Autodesk Inventor part; units mm, degrees
ref_plane "YZ Plane" through (0, 0, 0) normal (1, 0, 0) x (0, 1, 0)
ref_plane "XZ Plane" through (0, 0, 0) normal (0, 1, 0) x (-1, 0, 0)
ref_plane "XY Plane" through (0, 0, 0) normal (0, 0, 1) x (1, 0, 0)
sketch "Sketch1" plane through (0, 0, 0) normal (0, 0, 1) x (1, 0, 0)
  line L0 (6.4658, -12.7) -> (12.7, -12.7)
  arc A0 (-6.4658, -12.7) -> (6.4658, -12.7) centre (0, 0) ccw
  line L1 (-12.7, -12.7) -> (-6.4658, -12.7)
  line L2 (-12.7, -6.4658) -> (-12.7, -12.7)
  arc A1 (-12.7, 6.4658) -> (-12.7, -6.4658) centre (0, 0) ccw
  line L3 (-12.7, 12.7) -> (-12.7, 6.4658)
  line L4 (-6.4658, 12.7) -> (-12.7, 12.7)
  arc A2 (6.4658, 12.7) -> (-6.4658, 12.7) centre (0, 0) ccw
  line L5 (12.7, 12.7) -> (6.4658, 12.7)
  line L6 (12.7, 6.4658) -> (12.7, 12.7)
  arc A3 (12.7, -6.4658) -> (12.7, 6.4658) centre (0, 0) ccw
  line L7 (12.7, -12.7) -> (12.7, -6.4658)
  arc A4 (22.4506, 22.4506) -> (11.1037, -29.7451) centre (0, 0) ccw
  line L8 (53.8815, -8.9803) -> (157.065, -121.1361)
  line L9 (157.065, -121.1361) -> (447.7579, -29.481)
  line L10 (157.065, -121.1361) -> (461.865, -121.1361) construction
  circle A5 centre (463.0337, -77.9298) radius 50.8
  circle A6 centre (419.3415, -191.752) radius 50.8
  line L11 (463.0337, -77.9298) -> (419.3415, -191.752)
  line L12 (463.0337, -77.9298) -> (584.9537, -77.9298) construction
  arc A7 (-31.41, -4.6344) -> (323.0536, -260.3138) centre (270.1256, 39.8556) ccw
  line L13 (428.1628, -241.7802) -> (323.0536, -260.3138)
  line L14 (428.1628, -241.7802) -> (534.8936, -241.7802) construction
  line L15 (510.4596, -96.1349) -> (466.7674, -209.9571)
  circle A8 centre (0, -19.05) radius 2
  circle A9 centre (19.05, 0) radius 2
  circle A10 centre (-19.05, 0) radius 2
  circle A11 centre (0, 19.05) radius 2
  line L16 (22.4506, 22.4506) -> (53.8815, -8.9803)
  line L17 (52.7468, -14.1998) -> (11.1037, -29.7451)
  arc A12 (52.7468, -14.1998) -> (53.8815, -8.9803) centre (51.6365, -11.2253) ccw
  circle A13 centre (0, -19.05) radius 2.735
  circle A14 centre (-19.05, 0) radius 2.735
  circle A15 centre (0, 19.05) radius 2.735
  circle A16 centre (19.05, 0) radius 2.735
  circle A17 centre (463.0337, -77.9298) radius 25.4
  circle A18 centre (419.3415, -191.752) radius 25.4
  point P0 (50.8347, -14.9136)
  point P1 (54.0605, -9.1748)
  dimension "d0" = 152.4
  dimension "d1" = 304.8
  dimension "d2" = 17.5
  dimension "d3" = 101.6
  dimension "d4" = 101.6
  dimension "d5" = 121.92
  dimension "d6" = 111
  dimension "d7" = 609.6
  dimension "d9" = 170
  dimension "d10" = 4
  dimension "d11" = 4
  dimension "d12" = 4
  dimension "d13" = 4
  dimension "d16" = 50.8
  dimension "d17" = 50.8
extrude "Extrusion1" add sketch "Sketch1" along normal blind 3.175 contours L16 L8 L9 A5 L11 A6 L13 A7 A4 | A6 | A5 | A6 L11 A5 L15 | A13 | A14 | A15 | A16
fillet "Fillet1" radius 203.2 1 edges at (157.065, -121.1361, 1.5875)
properties part number "WhipperArm" material "MDF Medium Density Fiberboard"
The listing builds one solid part. Answer for the finished solid, in the listing's coordinates (mm). A direction names the side the tool comes from. Give positions to 0.01 mm unless a question says otherwise; leave off trailing zeros. Order: outer loops, then holes, each group sorted by start corner. A loop starts at its lowest first (then second) coordinate and runs counter-clockwise, first axis right, second up. Notation, with made-up numbers: (-17, -4) -> (41, -4) arc R6 cw to (41, 5) -> close; hole circle Ø3 at (-23, -4.5). An arc over 180 degrees is marked (long way). Put each result on its own line as item: value.
Item 1: Straight lines are drawn through the part: line 1 (Y direction, x = 19.05, z = 1.15); line 2 (X direction, y = -235, z = 2.55); line 3 (Y direction, x = 182, z = 1.7). For each, find the intervals that lie inside material, in ascending order.
Established:
line 1: y = -132.96 to -2, 2 to 25.4
line 2: x = 138.38 to 445.99
line 3: y = -251.93 to -88.27
Item 2: For a pull along Y with two mould halves and no side action, classify faces 3 (the face through (451.936, -230.717, 1.565)), 4 (the face through (237, -147, 0)), 5 (the face through (487.26, -85.56, 1.57)), 6 (the face through (165.2, -84.406, 1.61)) as released by +Y, released by -Y, zero draft, split by the parting line, or undercut.
Established:
face 3: released by -Y
face 4: zero draft
face 5: undercut
face 6: released by +Y
Item 3: For faces 1 (the face through (362.83, -56.26, 1.57)), 2 (the face through (393.966, -192.869, 1.565)), determine the directions among +Z, -Z, +X, -X, +Y, -Y from which every point of the face is accessible in a straight line to the end or side of a thin tool.
Established:
face 1: +Z, -Z, +Y
face 2: +Z, -Z
Item 4: A cutting plane is placed at D-D on x = 115.5. Give the vertices of the cut face in (y, z) (3 decimals), plus the area to 3 significant figures.
Established:
outline: (-222.811, 0) -> (-63.275, 0) -> (-63.275, 3.175) -> (-222.811, 3.175) -> close
area: 507 mm^2
Item 5: A cutting plane is placed at A-A on x = 406. Give the vertices of the cut face in (y, z) (3 decimals).
Established:
outline: (-245.688, 0) -> (-213.366, 0) -> (-213.366, 3.175) -> (-245.688, 3.175) -> close; (-170.138, 0) -> (-42.647, 0) -> (-42.647, 3.175) -> (-170.138, 3.175) -> close
Item 6: A cutting plane is placed at C-C on y = -114.5. Give the vertices of the cut face in (x, z) (3 decimals).
Established:
outline: (7.3, 0) -> (503.41, 0) -> (503.41, 3.175) -> (7.3, 3.175) -> close
Item 7: A cutting plane is placed at B-B on z = 1.3. Give the vertices of the cut face in (x, y).
Established:
outline: (-31.41, -4.63) arc R304.8 ccw to (323.05, -260.31) -> (428.16, -241.78) arc R50.8 ccw to (466.77, -209.96) -> (510.46, -96.13) arc R50.8 ccw to (447.76, -29.48) -> (280.26, -82.29) arc R203.2 cw to (69.61, -26.08) -> (53.88, -8.98) -> (22.45, 22.45) arc R31.75 ccw to start; hole circle Ø4 at (-19.05, 0); hole (-12.7, -12.7) -> (-6.47, -12.7) arc R14.25 ccw to (6.47, -12.7) -> (12.7, -12.7) -> (12.7, -6.47) arc R14.25 ccw to (12.7, 6.47) -> (12.7, 12.7) -> (6.47, 12.7) arc R14.25 ccw to (-6.47, 12.7) -> (-12.7, 12.7) -> (-12.7, 6.47) arc R14.25 ccw to (-12.7, -6.47) -> close; hole circle Ø4 at (0, -19.05); hole circle Ø4 at (0, 19.05); hole circle Ø4 at (19.05, 0); hole circle Ø50.8 at (419.34, -191.75); hole circle Ø50.8 at (463.03, -77.93)
Item 8: Given P1, Ø1.5, axis at y = -107, z = 1, coming from the +X side; P2, Ø1.6, axis at x = 9, z = 1.5, coming from the -Y side; P3, Ø3, axis at x = 0, y = -19.05, coming from the +Z side; P4, Ø1, axis at y = -42, z = 1.5, coming from the +X side, each flat-ended and moving along its own axis, determine where each tip first touches the part or whether it passes through.
Established:
P1: stops at x = 506.58
P2: stops at y = -118.68
P3: passes through
P4: stops at x = 499.44
